Geometry check sheet. Reference: the model listing, model coordinates, mm. A direction names the side the tool comes from. Round coordinates to 2 decimals unless told otherwise and drop trailing zeros. Order: outer loops, then holes, each group sorted by start corner. A loop starts at its lowest first (then second) coordinate and runs counter-clockwise, first axis right, second up.
Autodesk Inventor part; units mm, degrees
ref_plane "YZ Plane" through (0, 0, 0) normal (1, 0, 0) x (0, 1, 0)
ref_plane "XZ Plane" through (0, 0, 0) normal (0, 1, 0) x (-1, 0, 0)
ref_plane "XY Plane" through (0, 0, 0) normal (0, 0, 1) x (1, 0, 0)
sketch "Sketch1" plane through (0, 0, 0) normal (1, 0, 0) x (0, 1, 0)
  line L0 (-6, -12.5) -> (-6, -12.9)
  arc A0 (-6, -12.9) -> (-5.6, -13.3) centre (-5.6, -12.9) ccw
  line L1 (-5.6, -13.3) -> (-4.9, -13.3)
  arc A1 (-4.9, -13.3) -> (-4.7, -13.1) centre (-4.9, -13.1) ccw
  line L2 (-4.7, -13.1) -> (-4.7, -12.85)
  arc A2 (-4.5, -12.65) -> (-4.7, -12.85) centre (-4.5, -12.85) ccw
  line L3 (-4.5, -12.65) -> (-1.8, -12.65)
  arc A3 (-1.4, -13.05) -> (-1.8, -12.65) centre (-1.8, -13.05) ccw
  line L4 (-1.4, -13.05) -> (-1.4, -18.75)
  line L5 (-1.8, -19.15) -> (-4.5, -19.15)
  arc A4 (-1.8, -19.15) -> (-1.4, -18.75) centre (-1.8, -18.75) ccw
  arc A5 (-4.7, -18.95) -> (-4.5, -19.15) centre (-4.5, -18.95) ccw
  line L6 (-4.7, -18.95) -> (-4.7, -18.7)
  arc A6 (-4.7, -18.7) -> (-4.9, -18.5) centre (-4.9, -18.7) ccw
  line L7 (-4.9, -18.5) -> (-5.6, -18.5)
  arc A7 (-5.6, -18.5) -> (-6, -18.9) centre (-5.6, -18.9) ccw
  line L8 (-6, -18.9) -> (-6, -19.5)
  line L9 (-6.5, -6.5) -> (-6.5, -12.5)
  line L10 (-6.5, -12.5) -> (-2.5, -12.5)
  line L11 (-1.05, -19.5) -> (-6.5, -19.5)
  line L12 (-6.5, -19.5) -> (-6.5, -26)
  line L13 (-6.5, -26) -> (-1.05, -26)
  line L14 (-6, -26) -> (-6, -26.6)
  arc A8 (-6, -26.6) -> (-5.6, -27) centre (-5.6, -26.6) ccw
  line L15 (-5.6, -27) -> (-4.9, -27)
  arc A9 (-4.9, -27) -> (-4.7, -26.8) centre (-4.9, -26.8) ccw
  arc A10 (-4.5, -26.35) -> (-4.7, -26.55) centre (-4.5, -26.55) ccw
  line L16 (-4.7, -26.8) -> (-4.7, -26.55)
  line L17 (-4.5, -26.35) -> (-1.8, -26.35)
  arc A11 (-1.4, -26.75) -> (-1.8, -26.35) centre (-1.8, -26.75) ccw
  line L18 (-1.4, -26.75) -> (-1.4, -32.45)
  arc A12 (-1.8, -32.85) -> (-1.4, -32.45) centre (-1.8, -32.45) ccw
  line L19 (-1.8, -32.85) -> (-4.5, -32.85)
  arc A13 (-4.7, -32.65) -> (-4.5, -32.85) centre (-4.5, -32.65) ccw
  line L20 (-4.7, -32.65) -> (-4.7, -32.4)
  arc A14 (-4.7, -32.4) -> (-4.9, -32.2) centre (-4.9, -32.4) ccw
  line L21 (-4.9, -32.2) -> (-5.6, -32.2)
  arc A15 (-5.6, -32.2) -> (-6, -32.6) centre (-5.6, -32.6) ccw
  line L22 (-6, -32.6) -> (-6, -33)
  line L23 (-2.5, -33) -> (-6.5, -33)
  line L24 (-6.5, -33) -> (-6.5, -39)
  line L25 (32.5, 0) -> (0, 0)
  circle A16 centre (0, -6.5) radius 4.75
  circle A17 centre (32.5, -6.5) radius 4.75
  circle A18 centre (0, -39) radius 4.75
  circle A19 centre (32.5, -39) radius 4.75
  line L26 (39, -26) -> (39, -19.5)
  line L27 (39, -12.5) -> (39, -6.5)
  line L28 (39, -39) -> (39, -33)
  line L29 (26.5, -45.5) -> (32.5, -45.5)
  line L30 (0, -45.5) -> (6, -45.5)
  line L31 (13, -45.5) -> (19.5, -45.5)
  circle A20 centre (16.25, -22.75) radius 15
  circle A21 centre (16.2588, 5.0016) radius 2.5
  circle A22 centre (16.25, -50.5) radius 2.5
  circle A23 centre (16.25, -22.75) radius 5
  circle A24 centre (16.25, -22.75) radius 8.45
  line L32 (24.75, -27.6575) -> (24.75, -17.8425)
  line L33 (44, 10) -> (-11.5, 10)
  line L34 (-11.5, 10) -> (-11.5, -55.5)
  line L35 (-11.5, -55.5) -> (44, -55.5)
  line L36 (44, -55.5) -> (44, 10)
  line L37 (-11.5, 30) -> (44, 30)
  line L38 (-11.5, -75.5) -> (-11.5, 30)
  line L39 (44, 30) -> (44, -75.5)
  line L40 (44, -75.5) -> (-11.5, -75.5)
  circle A25 centre (16.25, -65.5) radius 5
  circle A26 centre (16.25, 20) radius 5
  arc A27 (11.25, -55.5) -> (21.25, -55.5) centre (16.25, -55.5) ccw
  line L41 (21.25, 10) -> (21.25, -55.5)
  line L42 (11.25, -55.5) -> (11.25, 10)
  arc A28 (21.25, 10) -> (11.25, 10) centre (16.25, 10) ccw
  line L43 (21.25, -45.5) -> (11.25, -45.5)
  point P0 (21.25, 0)
  point P1 (11.25, 0)
extrude "Extrusion1" add sketch "Sketch1" along normal blind 10 contours L41 A20 L42 L25 | L41 A24 L42 A20 | L41 A23 L42 A24 | L42 A24 L41 A20 | A20 L41 L43 L31 L42 | A23 | L41 A24 L42 A23
extrude "Extrusion2" add sketch "Sketch1" along normal blind 5 contours L25 L42 L33 L41 | L43 L31 L41 L35 L42
sketch "Sketch4" plane through (10, 21.25, 0) normal (0, 1, 0) x (1, 0, 0)
  line L0 (0, 45.5) -> (0, 0)
  circle A0 centre (0, 22.75) radius 2.5
  point P0 (-10, 0)
  dimension "d7" = 5
extrude "Extrusion4" cut sketch "Sketch4" against normal blind 10
properties part number "Cuchilla"
(1) Set-up check for faces 5 (the flat face through (5, 14, 7)), 6 (the flat face through (10, 16, -10)), 7 (the flat face through (7, 16, -45.5)): record each of +Z, -Z, +X, -X, +Y, -Y from which the full face is reachable in a straight line by a thin tool's end or side.
Returned:
face 5: +Z, +X, +Y, -Y
face 6: +Z, -Z, +X, +Y, -Y
face 7: -Z, +X, +Y, -Y
(2) Draft check along Z on faces 1 (the flat face through (7, 16, 0)), 2 (the flat face through (5, 15, -48)), 3 (the cylindrical face through (2.465, 13.752, -50.61)), 4 (the flat face through (2, 16, -55.5)). Enter one of: released by +Z, released by -Z, zero draft, split by the parting line, or undercut.
Returned:
face 1: released by +Z
face 2: zero draft
face 3: undercut
face 4: released by -Z
(3) Sectioned sample at B-B, the plane y = 16.25. Record the cut outline in (x, z), and give its area (3 significant figures).
Returned:
outline: (0, -55.5) - (5, -55.5) - (5, -53) - (0, -53) - close; (0, -48) - (5, -48) - (5, -45.5) - (10, -45.5) - (10, -25.25) arc R2.5 cw to (10, -20.25) - (10, 0) - (5, 0) - (5, 2.5) - (0, 2.5) - close; (0, 7.5) - (5, 7.5) - (5, 10) - (0, 10) - close
area: 495 mm2
(4) Sectioned sample at A-A, the plane x = 8.75. Record the cut outline in (y, z).
Returned:
outline: (11.25, -45.5) - (21.25, -45.5) - (21.25, -24.92) - (11.25, -24.92) - close; (11.25, -20.58) - (21.25, -20.58) - (21.25, 0) - (11.25, 0) - close
(5) Depth check by flat-ended pin: P1, Ø4, axis at x = 7.5, y = 18, coming from the -Z side; P2, Ø4, axis at x = 8, y = 18, coming from the +Z side; P3, Ø4, axis at y = 16.26, z = 5, coming from the -X side; P4, Ø3, axis at y = 18, z = 6.5, coming from the +X side. Enter the tip coordinate at first touch or a pass-through.
Returned:
P1: stops at z = -45.5
P2: stops at z = 0
P3: passes through
P4: stops at x = 5
(6) Material ranges on line 1 (Z direction, x = 2.55, y = 16.25); line 2 (Z direction, x = 1, y = 15); line 3 (Z direction, x = 6, y = 12.5), recorded low to high.
Returned:
line 1: z = -55.5 to -53, -48 to 2.5, 7.5 to 10
line 2: z = -55.5 to -52.67, -48.33 to 2.84, 7.16 to 10
line 3: z = -45.5 to 0
(7) Sectioned sample at D-D, the plane y = 12.25. Record the cut outline in (x, z).
Returned:
outline: (0, -55.5) - (5, -55.5) - (5, -45.5) - (10, -45.5) - (10, -25.25) arc R2.5 cw to (10, -20.25) - (10, 0) - (5, 0) - (5, 10) - (0, 10) - close
(8) Sectioned sample at C-C, the plane z = -22.75. Record the cut outline in (x, y).
Returned:
outline: (0, 11.25) - (7.5, 11.25) - (7.5, 21.25) - (0, 21.25) - close
